Read the model definition and answer for the solid it produces. Units are mm, in the model's axes. A direction names the side the tool comes from. Coordinates: 2 decimals unless noted, no trailing zeros. Loops run counter-clockwise (first coordinate to the right, second up) from the corner with the lowest first, then second, coordinate; pieces in that order, holes last.
from build123d import *

# Parameters (mm, degrees)
SKETCH1_W           = 68
SKETCH1_H           = 6
BOSS_EXTRUDE1_DEPTH = 124
BOSS_EXTRUDE2_DEPTH = 68
SKETCH4_W           = 68
SKETCH4_H           = 5.93639456
BOSS_EXTRUDE3_DEPTH = 68


with BuildPart() as part:
    # Sketch1 → Boss-Extrude1 (new body)
    with BuildSketch(Plane(origin=(0, 0, 0), x_dir=(1, 0, 0), z_dir=(0, 1, 0))):
        with Locations((34, 3)):
            Rectangle(SKETCH1_W, SKETCH1_H)
    extrude(amount=BOSS_EXTRUDE1_DEPTH)

    # Sketch3 → Boss-Extrude2 (add)
    with BuildSketch(Plane(origin=(0, 0, 0), x_dir=(0, 0, -1), z_dir=(1, 0, 0))):
        Polygon((0, 0), (-74.536565036, -13.142807465), (-72.911197136, -16.77309274), (6, 0), align=None)
    extrude(amount=BOSS_EXTRUDE2_DEPTH)

    # Sketch4 → Boss-Extrude3 (add)
    with BuildSketch(Plane.XY):
        with Locations((34, 121.03180272)):
            Rectangle(SKETCH4_W, SKETCH4_H)
    extrude(amount=BOSS_EXTRUDE3_DEPTH)


solid = part.part
Item 1: A cutting plane is placed at C-C on z = 8. Determine the outline of the cut face in (x, y), then the cut area to 3 significant figures.
Numbers:
outline: (0, -2.98) - (68, -2.98) - (68, -1.41) - (0, -1.41) - close; (0, 118.06) - (68, 118.06) - (68, 124) - (0, 124) - close
area: 510 mm2
Item 2: A cutting plane is placed at A-A on z = 60. Determine the outline of the cut face in (x, y).
Numbers:
outline: (0, -14.03) - (68, -14.03) - (68, -10.58) - (0, -10.58) - close; (0, 118.06) - (68, 118.06) - (68, 124) - (0, 124) - close
Item 3: Which of the six approach directions +Z, -Z, +X, -X, +Y, -Y give full straight-line access (tool end or side, diameter ignored) to faces 4 (the face through (33.52, -6.48, 36.75)), 5 (the face through (0, 69, -2)), 6 (the face through (34, 121, 68))?
Numbers:
face 4: +Z, +X, -X
face 5: +Z, -Z, -X, +Y, -Y
face 6: +Z, +X, -X, +Y
Item 4: Given pin 1 (2 mm diameter, centred on x = 42.5, z = 50, fed in from -Y); pin 2 (1 mm diameter, centred on x = 14, z = 66, fed in from -Y); pin 3 (12 mm diameter, centred on x = 51.5, z = 39.5, fed in from -Y); pin 4 (4 mm diameter, centred on y = 58.5, z = 3, fed in from -X), each flat-ended and moving along its own axis, determine where each tip first touches the part or whether it passes through.
Numbers:
pin 1: stops at y = -12.12
pin 2: stops at y = -15.41
pin 3: stops at y = -10.95
pin 4: passes through
Item 5: Find the intervals of material crossed by line 1 along Z through (x, y) = (52, 6); line 2 along Y through (x, z) = (29, 43.5); line 3 along Y through (x, z) = (57, 20), in increasing order.
Numbers:
line 1: z = -6 to 0
line 2: y = -10.52 to -7.67, 118.06 to 124
line 3: y = -5.53 to -3.53, 118.06 to 124
Item 6: A cutting plane is placed at D-D on y = 25. Determine the outline of the cut face in (x, z).
Numbers:
outline: (0, -6) - (68, -6) - (68, 0) - (0, 0) - close
Item 7: A cutting plane is placed at B-B on x = 42. Determine the outline of the cut face in (y, z).
Numbers:
outline: (-16.77, 72.91) - (0, -6) - (124, -6) - (124, 68) - (118.06, 68) - (118.06, 0) - (0, 0) - (-13.14, 74.54) - close
Item 8: Determine the mould class of faces 1 (the face through (34, 61, -6)), 2 (the face through (33.524, -8.504, 34.008)), 3 (the face through (34, 118.064, 34)) for opening direction Y: released by +Y, released by -Y, zero draft, split by the parting line, or undercut.
Numbers:
face 1: zero draft
face 2: released by -Y
face 3: undercut
